Design review of the part built by this model. Coordinates are the model's own, in mm. A direction names the side the tool comes from. Give positions to 0.01 mm unless a question says otherwise; leave off trailing zeros. Order: outer loops, then holes, each group sorted by start corner. A loop starts at its lowest first (then second) coordinate and runs counter-clockwise, first axis right, second up.
```python
from build123d import *

# Parameters (mm, degrees)
SKETCH1_R                = 4.1
BOSS_EXTRUDE1_DEPTH      = 3.5
BOSS_EXTRUDE2_DEPTH      = 51.7
BOSS_EXTRUDE2_DEPTH_BACK = 3.5
CHAMFER2_SIZE            = 5
CUT_EXTRUDE1_REACH       = 112.079
SKETCH4_W                = 51.7
SKETCH4_H                = 45
BOSS_EXTRUDE3_START      = 3.5
SKETCH5_R                = 4.1
BOSS_EXTRUDE3_DEPTH      = 3.5
CUT_EXTRUDE3_REACH       = 104.062
SKETCH9_R                = 1.35
SKETCH10_W               = 58.7
SKETCH10_H               = 53
BOSS_EXTRUDE5_DEPTH      = 3.175
SKETCH26_R               = 7.1
CUT_EXTRUDE6_DEPTH       = 4
SKETCH27_W               = 3.175
SKETCH27_H               = 34.600130378
BOSS_EXTRUDE6_DEPTH      = 45.22
SKETCH29_R               = 4.1
BOSS_EXTRUDE8_DEPTH      = 5.5
CHAMFER3_SIZE            = 3.175
BOSS_EXTRUDE9_START      = 10
SKETCH30_R               = 8
SKETCH30_R_2             = 4.1
BOSS_EXTRUDE9_DEPTH      = 10
SKETCH31_R               = 0.95
CUT_EXTRUDE7_DEPTH       = 120.972242206
BOSS_EXTRUDE10_DEPTH     = 45.22
SKETCH33_W               = 5.386290257
SKETCH33_H               = 2.7
BOSS_EXTRUDE11_DEPTH     = 45.22
BOSS_EXTRUDE12_DEPTH     = 0.2
SKETCH35_R               = 1.35
CUT_EXTRUDE8_DEPTH       = 5


with BuildPart() as part:
    # Sketch1 → Boss-Extrude1 (new body)
    with BuildSketch(Plane(origin=(0, 0, 0), x_dir=(0, 0, -1), z_dir=(1, 0, 0))):
        with BuildLine():
            Line((-17.5, 0), (-17.5, -20))
            Line((-17.5, -20), (-22.5, -20))
            Line((-22.5, -20), (-22.5, -76))
            Line((-22.5, -76), (22.5, -76))
            Line((22.5, -76), (22.5, -20))
            Line((22.5, -20), (17.5, -20))
            Line((17.5, -20), (17.5, 0))
            ThreePointArc((17.5, 0), (0, 17.5), (-17.5, 0))
        make_face()
        Circle(SKETCH1_R, mode=Mode.SUBTRACT)
    extrude(amount=-BOSS_EXTRUDE1_DEPTH)

    # Sketch2 → Boss-Extrude2 (add, two sides: drawn at the far end of the back side and taken through both)
    with BuildSketch(Plane(origin=(0, 0, 0), x_dir=(0, 0, -1), z_dir=(1, 0, 0)).offset(-BOSS_EXTRUDE2_DEPTH_BACK)):
        Polygon((-22.5, -20), (-22.5, -76), (22.5, -76), (22.5, -20), (26.5, -20), (26.5, -79.175), (-26.5, -79.175), (-26.5, -20), align=None)
    extrude(amount=BOSS_EXTRUDE2_DEPTH + BOSS_EXTRUDE2_DEPTH_BACK)

    # Chamfer2
    chamfer2_edges = [part.edges().sort_by_distance(p)[0] for p in [
        (24.1, -20, -26.5),
        (24.1, -20, 26.5),
    ]]
    chamfer(chamfer2_edges, length=CHAMFER2_SIZE)

    # Sketch4 → Cut-Extrude1 (cut, up to next)
    with BuildSketch(Plane(origin=(0, -76, 0), x_dir=(1, 0, 0), z_dir=(0, 1, 0)), mode=Mode.PRIVATE) as cut_extrude1_sk1:
        with Locations((25.85, 0)):
            Rectangle(SKETCH4_W, SKETCH4_H)
    cut_extrude1_tool1 = extrude(cut_extrude1_sk1.sketch, amount=-CUT_EXTRUDE1_REACH, mode=Mode.PRIVATE) & part.part
    add(cut_extrude1_tool1.solids().sort_by_distance((25.85, -76, 0))[0], mode=Mode.SUBTRACT)

    # Sketch5 → Boss-Extrude3 (add)
    with BuildSketch(Plane(origin=(51.7, 0, 0), x_dir=(0, 0, -1), z_dir=(1, 0, 0)).offset(BOSS_EXTRUDE3_START)):
        with BuildLine():
            Line((21.5, -20), (17.5, -20))
            Line((17.5, -20), (17.5, 0))
            ThreePointArc((17.5, 0), (0, 17.5), (-17.5, 0))
            Line((-17.5, 0), (-17.5, -20))
            Line((-17.5, -20), (-21.5, -20))
            Line((-21.5, -20), (-26.5, -25))
            Line((-26.5, -25), (-26.5, -79.175))
            Line((-26.5, -79.175), (26.5, -79.175))
            Line((26.5, -79.175), (26.5, -25))
            Line((26.5, -25), (21.5, -20))
        make_face()
        Circle(SKETCH5_R, mode=Mode.SUBTRACT)
    extrude(amount=-BOSS_EXTRUDE3_DEPTH)

    # Sketch9 → Cut-Extrude3 (cut, up to next)
    with BuildSketch(Plane(origin=(55.2, 0, 0), x_dir=(0, 0, -1), z_dir=(1, 0, 0)), mode=Mode.PRIVATE) as cut_extrude3_sk1:
        with Locations((0, 8.125)):
            Circle(SKETCH9_R)
    cut_extrude3_tool1 = extrude(cut_extrude3_sk1.sketch, amount=-CUT_EXTRUDE3_REACH, mode=Mode.PRIVATE) & part.part
    # Sketch9 → Cut-Extrude3 (cut, up to next)
    with BuildSketch(Plane(origin=(55.2, 0, 0), x_dir=(0, 0, -1), z_dir=(1, 0, 0)), mode=Mode.PRIVATE) as cut_extrude3_sk2:
        with Locations((8.125, 0)):
            Circle(SKETCH9_R)
    cut_extrude3_tool2 = extrude(cut_extrude3_sk2.sketch, amount=-CUT_EXTRUDE3_REACH, mode=Mode.PRIVATE) & part.part
    # Sketch9 → Cut-Extrude3 (cut, up to next)
    with BuildSketch(Plane(origin=(55.2, 0, 0), x_dir=(0, 0, -1), z_dir=(1, 0, 0)), mode=Mode.PRIVATE) as cut_extrude3_sk3:
        with Locations((0, -8.125)):
            Circle(SKETCH9_R)
    cut_extrude3_tool3 = extrude(cut_extrude3_sk3.sketch, amount=-CUT_EXTRUDE3_REACH, mode=Mode.PRIVATE) & part.part
    # Sketch9 → Cut-Extrude3 (cut, up to next)
    with BuildSketch(Plane(origin=(55.2, 0, 0), x_dir=(0, 0, -1), z_dir=(1, 0, 0)), mode=Mode.PRIVATE) as cut_extrude3_sk4:
        with Locations((-8.125, 0)):
            Circle(SKETCH9_R)
    cut_extrude3_tool4 = extrude(cut_extrude3_sk4.sketch, amount=-CUT_EXTRUDE3_REACH, mode=Mode.PRIVATE) & part.part
    add(cut_extrude3_tool1.solids().sort_by_distance((55.2, 8.125, 0))[0], mode=Mode.SUBTRACT)
    add(cut_extrude3_tool2.solids().sort_by_distance((55.2, 0, -8.125))[0], mode=Mode.SUBTRACT)
    add(cut_extrude3_tool3.solids().sort_by_distance((55.2, -8.125, 0))[0], mode=Mode.SUBTRACT)
    add(cut_extrude3_tool4.solids().sort_by_distance((55.2, 0, 8.125))[0], mode=Mode.SUBTRACT)

    # Sketch10 → Boss-Extrude5 (add)
    with BuildSketch(Plane.XZ.offset(79.175)):
        with Locations((25.85, 0)):
            Rectangle(SKETCH10_W, SKETCH10_H)
    extrude(amount=BOSS_EXTRUDE5_DEPTH)

    # Sketch26 → Cut-Extrude6 (cut)
    with BuildSketch(Plane.XY.offset(26.5)):
        with Locations((25.85, -69.065)):
            Circle(SKETCH26_R)
    extrude(amount=-CUT_EXTRUDE6_DEPTH, mode=Mode.SUBTRACT)

    # Sketch27 → Boss-Extrude6 (add)
    with BuildSketch(Plane(origin=(0, -79.175, 0), x_dir=(1, 0, 0), z_dir=(0, 1, 0))):
        with Locations((39.993724488, -5.199934811)):
            Rectangle(SKETCH27_W, SKETCH27_H)
        with Locations((11.706275512, -5.199934811)):
            Rectangle(SKETCH27_W, SKETCH27_H)
    extrude(amount=BOSS_EXTRUDE6_DEPTH)

    # Sketch29 → Boss-Extrude8 (add)
    with BuildSketch(Plane(origin=(0, 0, -26.5), x_dir=(-1, 0, 0), z_dir=(0, 0, -1))):
        with BuildLine():
            Line((-40.997321429, -82.35), (-55.2, -82.35))
            Line((-55.2, -82.35), (-31.95, -117.07))
            ThreePointArc((-31.95, -117.07), (-25.85, -123.17), (-19.75, -117.07))
            Line((-19.75, -117.07), (3.5, -82.35))
            Line((3.5, -82.35), (-10.702678571, -82.35))
            Line((-10.702678571, -82.35), (-10.702678571, -88.35))
            Line((-10.702678571, -88.35), (-20.85, -103.503333333))
            Line((-20.85, -103.503333333), (-30.85, -103.503333333))
            Line((-30.85, -103.503333333), (-40.997321429, -88.35))
            Line((-40.997321429, -88.35), (-40.997321429, -82.35))
        make_face()
        with Locations(Location((-25.85, -117.07, 0), (0, 0, 90))):
            Circle(SKETCH29_R, mode=Mode.SUBTRACT)
    extrude(amount=-BOSS_EXTRUDE8_DEPTH)

    # Chamfer3
    chamfer3_edges = [part.edges().sort_by_distance(p)[0] for p in [
        (43.575, -99.71, -26.5),
        (8.125, -99.71, -26.5),
        (-3.5, -53.675, -26.5),
        (-3.5, -53.675, 26.5),
        (55.2, -53.675, 26.5),
        (55.2, -53.675, -26.5),
    ]]
    chamfer(chamfer3_edges, length=CHAMFER3_SIZE)

    # Sketch30 → Boss-Extrude9 (add)
    with BuildSketch(Plane(origin=(0, 0, 0), x_dir=(0, 0, -1), z_dir=(1, 0, 0)).offset(BOSS_EXTRUDE9_START)):
        Circle(SKETCH30_R)
        Circle(SKETCH30_R_2, mode=Mode.SUBTRACT)
    extrude(amount=-BOSS_EXTRUDE9_DEPTH)

    # Sketch31 → Cut-Extrude7 (cut, through all)
    with BuildSketch(Plane(origin=(0, -20, 0), x_dir=(1, 0, 0), z_dir=(0, 1, 0))):
        with Locations(Location((5, 0, 0), (0, 0, 90))):
            Circle(SKETCH31_R)
    extrude(amount=CUT_EXTRUDE7_DEPTH, mode=Mode.SUBTRACT)

    # Sketch32 → Boss-Extrude10 (add)
    with BuildSketch(Plane(origin=(0, -79.175, 0), x_dir=(1, 0, 0), z_dir=(0, 1, 0))):
        Polygon((13.293775512, 12.600036526), (16.4, 12.600036526), (16.4, 15.600130378), (10.118775512, 15.600130378), (10.118775512, 12.100130378), (13.293775512, 12.100130378), align=None)
    boss_extrude10 = extrude(amount=BOSS_EXTRUDE10_DEPTH)

    # Sketch33 → Boss-Extrude11 (add)
    with BuildSketch(Plane(origin=(0, -79.175, 0), x_dir=(1, 0, 0), z_dir=(0, 1, 0))):
        with Locations((15.986920641, -21.15)):
            Rectangle(SKETCH33_W, SKETCH33_H)
    boss_extrude11 = extrude(amount=BOSS_EXTRUDE11_DEPTH)

    # Mirror1: Boss-Extrude10, Boss-Extrude11 across plane
    add(boss_extrude10.mirror(Plane.ZY.offset(-25.85)))
    add(boss_extrude11.mirror(Plane.ZY.offset(-25.85)))

    # Sketch34 → Boss-Extrude12 (add)
    with BuildSketch(Plane(origin=(0, -33.955, 0), x_dir=(1, 0, 0), z_dir=(0, 1, 0))):
        Polygon((13.293775512, -19.8), (13.293775512, 12.600036526), (16.4, 12.600036526), (16.4, 15.600130378), (10.118775512, 15.600130378), (10.118775512, -22.5), (18.680065769, -22.5), (18.680065769, -19.8), align=None)
        Polygon((41.581224488, -22.5), (41.581224488, 15.600130378), (35.3, 15.600130378), (35.3, 12.600036526), (38.406224488, 12.600036526), (38.406224488, -19.8), (33.019934231, -19.8), (33.019934231, -22.5), align=None)
    extrude(amount=BOSS_EXTRUDE12_DEPTH)

    # Sketch35 → Cut-Extrude8 (cut)
    with BuildSketch(Plane.XY.offset(26.5)):
        with Locations((36.668603525, -39.204067417)):
            Circle(SKETCH35_R)
        with Locations((25.849997965, -39.204067417)):
            Circle(SKETCH35_R)
        with Locations((15.031392404, -39.204067417)):
            Circle(SKETCH35_R)
    extrude(amount=-CUT_EXTRUDE8_DEPTH, mode=Mode.SUBTRACT)


solid = part.part
```
1. Machinability: for faces 4 (the face through (29.13, -75.36, 24.53)), 5 (the face through (10.119, -57, 3)), 6 (the face through (53.47, 0.41, 6.84)), which of the approach directions +Z, -Z, +X, -X, +Y, -Y give a long, thin tool a straight path to every point of the face, cutting with its end or side? Answer none if there is none.
Recorded:
face 4: +Z
face 5: +Y
face 6: +X
2. For line 1 along X through (y, z) = (-77, 14); line 2 along Z through (x, y) = (13.5, -76.5); line 3 along X through (y, z) = (-75.5, -15), list the stretches that pass through material, from the lowest coordinate up.
Recorded:
line 1: x = -3.5 to 0, 10.12 to 13.29, 38.41 to 41.58, 51.7 to 55.2
line 2: z = -26.5 to -22.5, -15.6 to -12.6, 19.8 to 26.5
line 3: x = -3.5 to 0, 10.12 to 16.4, 35.3 to 41.58, 51.7 to 55.2
3. Take a section at C-C (z = 13). State the section outline as (x, y) points (3 decimals), then the cut area to 3 significant figures.
Recorded:
outline: (-3.5, -82.35) - (55.2, -82.35) - (55.2, 11.715) - (51.7, 11.715) - (51.7, -79.175) - (41.581, -79.175) - (41.581, -33.755) - (38.406, -33.755) - (38.406, -79.175) - (13.294, -79.175) - (13.294, -33.755) - (10.119, -33.755) - (10.119, -79.175) - (0, -79.175) - (0, 11.715) - (-3.5, 11.715) - close
area: 1,110 mm2
4. Take a section at A-A (y = -48.5). State the section outline as (x, z) points (3 decimals).
Recorded:
outline: (-3.5, -23.325) - (-0.325, -26.5) - (52.025, -26.5) - (55.2, -23.325) - (55.2, 23.325) - (52.025, 26.5) - (-0.325, 26.5) - (-3.5, 23.325) - close; hole (0, -22.5) - (51.7, -22.5) - (51.7, 22.5) - (41.581, 22.5) - (41.581, -15.6) - (35.3, -15.6) - (35.3, -12.6) - (38.406, -12.6) - (38.406, 19.8) - (33.02, 19.8) - (33.02, 22.5) - (18.68, 22.5) - (18.68, 19.8) - (13.294, 19.8) - (13.294, -12.6) - (16.4, -12.6) - (16.4, -15.6) - (10.119, -15.6) - (10.119, 22.5) - (0, 22.5) - close
5. Draft analysis for pull direction Z (two halves, no side actions). For faces 1 (the face through (-1.726, 17.496, -0.385)), 2 (the face through (-3.5, -32, 0)), 3 (the face through (41.581, -57, 3)), state which applies: pulls with the +Z half, pulls with the -Z half, needs draft (parallel to the pull), parting line crosses it, or undercut.
Recorded:
face 1: parting line crosses it
face 2: needs draft
face 3: undercut
6. For pin 1 (4.5 mm diameter, centred on x = 12.5, z = 11.5, fed in from +Y) (3 decimals); pin 2 (3 mm diameter, centred on y = -85.5, z = -23, fed in from +X); pin 3 (1.8 mm diameter, centred on x = -2.5, y = -15, fed in from -Z), all flat-tipped, find the tip position at first contact; note any pin that passes through.
Recorded:
pin 1: stops at y = -33.755
pin 2: stops at x = 54.1
pin 3: stops at z = -17.5
7. Take a section at B-B (x = 46). State the section outline as (y, z) points (3 decimals).
Recorded:
outline: (-96.089, -23.325) - (-90.382, -26.5) - (-25, -26.5) - (-21, -22.5) - (-79.175, -22.5) - (-79.175, 22.5) - (-21, 22.5) - (-25, 26.5) - (-82.35, 26.5) - (-82.35, -21) - (-96.089, -21) - close
